Check sheet for the modelled part. Datum: model origin and axes. Units: mm. A direction names the side the tool comes from. Coordinates: 2 decimals unless noted, no trailing zeros. Loops run counter-clockwise (first coordinate to the right, second up) from the corner with the lowest first, then second, coordinate; pieces in that order, holes last. Notation, with made-up numbers: (80.5, 79) - (126.5, 79) arc R28 ccw to (126.5, 111) - close; hole circle Ø10 at (20.25, -36). An arc over 180 degrees is marked (long way). Use a Markdown table: item, result. Add a question column.
1) Thickness scan on line 1 (Z direction, x = 99, y = -20.5); line 2 (Y direction, x = 12.5, z = 55); line 3 (Z direction, x = 10.5, y = 26) (3 decimals). Record the ranges inside material, lowest first.
2) Go/stop test with flat-tipped pins: P1, Ø6.5, axis at y = 16.5, z = 16.5, coming from the -X side (3 decimals); P2, Ø3, axis at x = 25.5, z = 12.5, coming from the -Y side; P3, Ø7.5, axis at x = 78.5, y = -10.5, coming from the -Z side. Record where each tip stops, or that it passes through.
3) Tool access check on faces 1 (the flat face through (52, -25.4, 43)), 2 (the cylindrical face through (36.393, 18.961, 52.776)), 3 (the cylindrical face through (115.03, -7.63, 55.76)), 4 (the flat face through (47.625, -1, 6)), 5 (the flat face through (71, -19, 45.046)). Record the directions out of +Z, -Z, +X, -X, +Y, -Y that give a thin tool (end or side, any length) a straight path to the whole face; none if there is none.
4) Sectioned sample at B-B, the plane y = -31.5. Enter the section's corners in (x, z) (3 decimals), then the cut area to 3 significant figures.
5) Sectioned sample at A-A, the plane x = 75. Enter the section's corners in (y, z), then the cut area to 3 significant figures.
from build123d import *

# Parameters (mm, degrees)
F1_DEPTH = 63.5
F2_DEPTH = 12.7
F0_W     = 25.4
F0_H     = 19.0624117216
F3_DEPTH = 25.4


# Not quite as in the source:
# - a feature names something its author has since deleted; it is built from what else it names


with BuildPart() as f1:
    # F0 (on Front) → F1 (new body, symmetric)
    with BuildSketch(Plane.XZ):
        Polygon((47.625, -9.525), (47.625, 9.525), (28.575, 9.525), (-47.625, 9.525), (-47.625, -9.525), align=None)
    extrude(amount=F1_DEPTH, both=True)

    # F0 (on Front) → F2 (join, symmetric)
    with BuildSketch(Plane.XZ):
        with BuildLine():
            Line((-47.625, 9.525), (28.575, 9.525))
            Line((28.575, 9.525), (28.575, 31.3774505112))
            ThreePointArc((28.575, 31.3774505112), (36.1870844323, 52.5292330788), (55.5320502217, 63.9797367269))
            add(Edge.make_bspline(
                [(-47.625, 9.525), (-32.001836586, 27.9945600123), (-8.2663538638, 59.5795130057), (42.691262939, 63.5782592588), (55.5320502217, 63.9797367269)],
                knots=[0, 0, 0, 0, 0.463039199, 0.7597377555, 0.7597377555, 0.7597377555, 0.7597377555], degree=3))
        make_face()
    extrude(amount=F2_DEPTH, both=True)

    # F0 (on Front) → F3 (join, symmetric)
    with BuildSketch(Plane.XZ):
        with BuildLine():
            Line((28.575, 9.525), (47.625, 9.525))
            Line((47.625, 9.525), (47.625, 31.3774505112))
            ThreePointArc((47.625, 31.3774505112), (53.1477549989, 42.5899481953), (65.4029340449, 45.0458622098))
            Line((65.4029340449, 45.0458622098), (65.4029340449, 64.1082739314))
            add(Edge.make_bspline(
                [(55.5320502217, 63.9797367269), (59.6889735266, 64.1097062534), (63.1060550499, 64.1180929217), (65.4029340449, 64.1082739314)],
                knots=[0.7597377555, 0.7597377555, 0.7597377555, 0.7597377555, 0.8557874071, 0.8557874071, 0.8557874071, 0.8557874071], degree=3))
            ThreePointArc((55.5320502217, 63.9797367269), (36.1870844323, 52.5292330788), (28.575, 31.3774505112))
            Line((28.575, 31.3774505112), (28.575, 9.525))
        make_face()
        with Locations((78.1029340449, 54.5770680706)):
            Rectangle(F0_W, F0_H)
    extrude(amount=F3_DEPTH, both=True)

    # F0 (on Front) → F4 (revolve)
    with BuildSketch(Plane.XZ):
        Polygon((90.8029340449, 64.1082739314), (90.8029340449, 45.0458622098), (90.8029340449, 38.931951193), (116.2029340449, 38.931951193), (116.2029340449, 72.13054624), (90.8029340449, 72.13054624), align=None)
    revolve(axis=Axis((90.8029340449, 0, 55.5312487165), (0, 0, -1)))


solid = f1.part
Solved:
| question | item | result |
|---|---|---|
| 1 | line 1 | z = 38.93 to 72.13 |
| 1 | line 2 | y = -12.7 to 12.7 |
| 1 | line 3 | z = -9.525 to 9.525 |
| 2 | P1 | stops at x = 28.575 |
| 2 | P2 | stops at y = -12.7 |
| 2 | P3 | stops at z = 38.93 |
| 3 | face 1 | +Z, +X, -X, -Y |
| 3 | face 2 | +Z, -X, +Y |
| 3 | face 3 | none |
| 3 | face 4 | -Z, +X, +Y, -Y |
| 3 | face 5 | -Z, -Y |
| 4 | outline | (-47.625, -9.525) - (47.625, -9.525) - (47.625, 9.525) - (-47.625, 9.525) - close |
| 4 | area | 1,810 mm2 |
| 5 | outline | (-25.4, 45.05) - (-19.89, 45.05) - (-19.89, 38.93) - (19.89, 38.93) - (19.89, 45.05) - (25.4, 45.05) - (25.4, 64.11) - (19.89, 64.11) - (19.89, 72.13) - (-19.89, 72.13) - (-19.89, 64.11) - (-25.4, 64.11) - close |
| 5 | area | 1,530 mm2 |
